The model under review builds one solid part; all positions refer to its coordinate system, in mm. A direction names the side the tool comes from. Give positions to 0.01 mm unless a question says otherwise; leave off trailing zeros. Order: outer loops, then holes, each group sorted by start corner. A loop starts at its lowest first (then second) coordinate and runs counter-clockwise, first axis right, second up. Notation, with made-up numbers: (3.5, 77.25) - (35.5, 77.25) arc R14 cw to (35.5, 97.25) - close; hole circle Ø3 at (25.5, 76.25). An arc over 180 degrees is marked (long way). Put each result on its own line as item: value.
Autodesk Inventor part; units mm, degrees
ref_plane "YZ Plane" through (0, 0, 0) normal (1, 0, 0) x (0, 1, 0)
ref_plane "XZ Plane" through (0, 0, 0) normal (0, 1, 0) x (-1, 0, 0)
ref_plane "XY Plane" through (0, 0, 0) normal (0, 0, 1) x (1, 0, 0)
sketch "スケッチ1" plane through (0, 0, 0) normal (0, 0, 1) x (1, 0, 0)
  circle A0 centre (0, 0) radius 1.4
  circle A1 centre (0, 0) radius 3
  dimension "d0" = 2.8
  dimension "d1" = 6
extrude "押し出し1" add sketch "スケッチ1" along normal blind 48 contours A0 | A1
sketch "スケッチ2" plane through (0, 0, 48) normal (0, 0, 1) x (1, 0, 0)
  circle A0 centre (0, 0) radius 1.4
  dimension "d4" = 2.8
extrude "押し出し2" cut sketch "スケッチ2" against normal blind 6
extrude "押し出し3" cut sketch "スケッチ1" along normal blind 6 contours A0
properties part number "40mm" material "アルミニウム 6061"
(1) Take a section at D-D, the plane y = 2.6. Write out the cut boundary in (x, z), then the cut area to 3 significant figures.
The answers:
outline: (-1.5, 0) - (1.5, 0) - (1.5, 48) - (-1.5, 48) - close
area: 144 mm^2
(2) Take a section at A-A, the plane x = 0. Write out the cut boundary in (y, z).
The answers:
outline: (-3, 0) - (-1.4, 0) - (-1.4, 6) - (1.4, 6) - (1.4, 0) - (3, 0) - (3, 48) - (1.4, 48) - (1.4, 42) - (-1.4, 42) - (-1.4, 48) - (-3, 48) - close
(3) Take a section at B-B, the plane z = 4. Write out the cut boundary in (x, y), then the cut area to 3 significant figures.
The answers:
outline: circle Ø6 at (0, 0); hole circle Ø2.8 at (0, 0)
area: 22.1 mm^2
(4) Wall thickness on L1, parallel to Y at x = 0, z = 1.75; L2, parallel to Z at x = -0.6, y = 0.55; L3, parallel to Y at x = -0.2, z = 38.5: over which ranges is each line inside the solid? List them lowest first.
The answers:
L1: -3 to -1.4, 1.4 to 3
L2: 6 to 42
L3: -2.99 to 2.99
(5) The part is to be moulded in two halves that separate along X. For faces 1 (the flat face through (0, 0, 6)), 2 (the flat face through (0, 0, 42)), 3 (the cylindrical face through (-3, 0, 24)), say which applies: pulls with the +X half, pulls with the -X half, needs draft (parallel to the pull), parting line crosses it, or undercut.
The answers:
face 1: undercut
face 2: undercut
face 3: parting line crosses it
(6) For faces 4 (the cylindrical face through (-1.4, -0.06, 2.96)), 5 (the cylindrical face through (-1.4, 0.06, 45.04)), list the 3-axis set-ups (+Z, -Z, +X, -X, +Y, -Y) from which the entire face can be reached by the end or side of a thin tool; tool diameter is ignored.
The answers:
face 4: -Z
face 5: +Z
(7) Take a section at C-C, the plane z = 10. Write out the cut boundary in (x, y), then the cut area to 3 significant figures.
The answers:
outline: circle Ø6 at (0, 0)
area: 28.3 mm^2
(8) Clearance check with flat-ended pins moving along their axes: pin 1 Ø1.5 at (x, z) = (2, 5.5) entering from -Y; pin 2 Ø3 at (x, y) = (0.5, -0.5) entering from +Z; pin 3 Ø2.5 at (x, y) = (0, 0) entering from +Z; pin 4 Ø2 at (y, z) = (2.5, 32.5) entering from +X. State where each tip first meets the part, or that it passes through.
The answers:
pin 1: y = -2.73
pin 2: z = 48
pin 3: z = 42
pin 4: x = 2.6
